Verification items for the finished model (mm, model axes). Coordinates: 2 decimals unless noted, no trailing zeros. Loops run counter-clockwise (first coordinate to the right, second up) from the corner with the lowest first, then second, coordinate; pieces in that order, holes last. Notation, with made-up numbers: (58, 19.25) - (70, 19.25) arc R12 ccw to (70, 26.25) - close; hole circle Ø8 at (-23.5, 29). An arc over 180 degrees is marked (long way). Answer as CSV lines item,"result". Start each with the question number.
1. Release check for a two-part mould opening along Y. For faces 1 (the cylindrical face through (-14.715, -14.699, 1.014)), 2 (the cylindrical face through (7.526, -10.648, 0.986)), 3 (the flat face through (-15, 0, 1)) record: pulls with the +Y half, pulls with the -Y half, needs draft (parallel to the pull), parting line crosses it, or undercut.
2. Material ranges on line 1 (Y direction, x = -9, z = 0.95); line 2 (X direction, y = -10.5, z = 1.85); line 3 (Y direction, x = -4.5, z = 0.4), recorded low to high. Write a range as [from, to].
3. Gauge pin test, flat end, axial feed: P1, Ø3, axis at x = 0, y = -5, coming from the -Z side. Record the tip position at first contact, or that the pin passes through.
4. Cross-section at B-B (x = -9). Enter the section's corners in (y, z), plus the area to 3 significant figures.
5. Cross-section at D-D (z = 1.15). Enter the section's corners in (x, y), plus the area to 3 significant figures.
6. Cross-section at C-C (x = -4.5). Enter the section's corners in (y, z), plus the area to 3 significant figures.
7. Cross-section at A-A (y = -12). Enter the section's corners in (x, z).
```python
from build123d import *

# Parameters (mm, degrees)
SKETCH_W  = 30
SKETCH_H  = 30
SKETCH_R  = 2
PAD_DEPTH = 2
FILLET_R  = 1


with BuildPart() as part:
    # Sketch → Pad (new body)
    with BuildSketch(Plane.XY):
        Rectangle(SKETCH_W, SKETCH_H)
        with Locations((-9, -12)):
            Circle(SKETCH_R, mode=Mode.SUBTRACT)
        with Locations((-9, -4)):
            Circle(SKETCH_R, mode=Mode.SUBTRACT)
        with Locations((9, -4)):
            Circle(SKETCH_R, mode=Mode.SUBTRACT)
        with Locations((9, -12)):
            Circle(SKETCH_R, mode=Mode.SUBTRACT)
        with Locations((0, -5)):
            Circle(SKETCH_R, mode=Mode.SUBTRACT)
        with Locations((4.5, 5)):
            Circle(SKETCH_R, mode=Mode.SUBTRACT)
        with Locations((-4.5, 5)):
            Circle(SKETCH_R, mode=Mode.SUBTRACT)
    extrude(amount=PAD_DEPTH)

    # Fillet
    fillet_edges = [part.edges().sort_by_distance(p)[0] for p in [
        (-15, -15, 1),
        (15, -15, 1),
        (-15, 15, 1),
        (15, 15, 1),
    ]]
    fillet(fillet_edges, radius=FILLET_R)


solid = part.part
```
Values follow:
1,face 1,"pulls with the -Y half"
1,face 2,"undercut"
1,face 3,"needs draft"
2,line 1,"y = [-15, -14], [-10, -6], [-2, 15]"
2,line 2,"x = [-15, -10.32], [-7.68, 7.68], [10.32, 15]"
2,line 3,"y = [-15, 3], [7, 15]"
3,P1,"passes through"
4,outline,"(-15, 0) - (-14, 0) - (-14, 2) - (-15, 2) - close; (-10, 0) - (-6, 0) - (-6, 2) - (-10, 2) - close; (-2, 0) - (15, 0) - (15, 2) - (-2, 2) - close"
4,area,"44.0 mm²"
5,outline,"(-15, -14) arc R1 ccw to (-14, -15) - (14, -15) arc R1 ccw to (15, -14) - (15, 14) arc R1 ccw to (14, 15) - (-14, 15) arc R1 ccw to (-15, 14) - close; hole circle Ø4 at (-9, -12); hole circle Ø4 at (-9, -4); hole circle Ø4 at (-4.5, 5); hole circle Ø4 at (0, -5); hole circle Ø4 at (4.5, 5); hole circle Ø4 at (9, -12); hole circle Ø4 at (9, -4)"
5,area,"811 mm²"
6,outline,"(-15, 0) - (3, 0) - (3, 2) - (-15, 2) - close; (7, 0) - (15, 0) - (15, 2) - (7, 2) - close"
6,area,"52.0 mm²"
7,outline,"(-15, 0) - (-11, 0) - (-11, 2) - (-15, 2) - close; (-7, 0) - (7, 0) - (7, 2) - (-7, 2) - close; (11, 0) - (15, 0) - (15, 2) - (11, 2) - close"
